For this review, take the finished solid that the model builds, in its own axes (mm). Coordinates: 2 decimals unless noted, no trailing zeros. Write each loop counter-clockwise with the first axis right and the second up, starting at its lowest first coordinate (ties: lowest second). Pieces come first, ordered by that corner, then holes. Notation, with made-up numbers: (28, -31.75) -> (40, -31.75) arc R35 cw to (40, 7.25) -> close; hole circle Ø4 at (-10, 65). An arc over 180 degrees is marked (long way). Put each result on its own line as item: value. Start each with the question number.
Item 1: Insertion check: P1, Ø1, axis at x = 56.5, y = 57, coming from the +Z side; P2, Ø2, axis at y = 45.5, z = 4.5, coming from the -X side; P3, Ø2, axis at x = -33.5, z = 5, coming from the -Y side; P4, Ø1.5, axis at y = 9.5, z = 1, coming from the +X side. Each pin has a flat end and moves straight along its axis. Give the tip position at first contact, or say it passes through.
Item 2: The part is to be moulded in two halves that separate along Y. For faces 1 (the flat face through (1, 75, 5)), 2 (the flat face through (18, 1, 0)), 3 (the cylindrical face through (75.092, 15.007, 5.055)), say which applies: +Y half, -Y half, draft (parallel to the pull), parting line (faces both ways), or undercut.
Item 3: Consider section A-A on z = 8.5. Give the boundary of the cut face in (x, y), and give its area (3 significant figures).
Item 4: Consider section B-B on x = 0. Give the boundary of the cut face in (y, z).
Item 5: To check wall thickness, follow L1, parallel to Y at x = 0, z = 4.25; L2, parallel to Y at x = -10, z = 0.5; L3, parallel to X at y = -10, z = 4.75. State the ranges of each line that lie inside material, in increasing order.
Item 6: Consider section C-C on y = -58.5. Give the boundary of the cut face in (x, z), and give its area (3 significant figures).
Item 7: Consider section D-D on x = 68. Give the boundary of the cut face in (y, z).
```python
from build123d import *

# Parameters (mm, degrees)
BOSS_EXTRUDE1_DEPTH = 10
SKETCH2_R           = 1.25
CUT_EXTRUDE1_DEPTH  = 5
CIRPATTERN1_COUNT   = 3
SKETCH3_R           = 15
CUT_EXTRUDE2_DEPTH  = 10


with BuildPart() as part:
    # Sketch1 → Boss-Extrude1 (new body)
    with BuildSketch(Plane.XY):
        Polygon((43.301270189, -75), (86.602540378, 0), (43.301270189, 75), (-43.301270189, 75), (-86.602540378, 0), (-43.301270189, -75), align=None)
    extrude(amount=BOSS_EXTRUDE1_DEPTH)

    # Sketch2 → Cut-Extrude1 (cut)
    with BuildSketch(Plane.XZ.offset(75)):
        with Locations((-33.301270189, 5)):
            Circle(SKETCH2_R)
        with Locations((-23.301270189, 5)):
            Circle(SKETCH2_R)
        with Locations(Location((33.301270189, 5, 0), (0, 0, 180))):
            Circle(SKETCH2_R)
        with Locations(Location((23.301270189, 5, 0), (0, 0, 180))):
            Circle(SKETCH2_R)
    cut_extrude1 = extrude(amount=-CUT_EXTRUDE1_DEPTH, mode=Mode.SUBTRACT)

    # CirPattern1: Cut-Extrude1 ×3 about axis
    cirpattern1_axis = Axis((0, 0, 0), (0, 0, 1))
    for i in range(1, CIRPATTERN1_COUNT):
        add(cut_extrude1.rotate(cirpattern1_axis, i * 360 / CIRPATTERN1_COUNT), mode=Mode.SUBTRACT)

    # Sketch3 → Cut-Extrude2 (cut)
    with BuildSketch(Plane.XY.offset(10)):
        Circle(SKETCH3_R)
    extrude(amount=-CUT_EXTRUDE2_DEPTH, mode=Mode.SUBTRACT)


solid = part.part
```
Return value:
1. P1: through
1. P2: x = -60.91
1. P3: y = -70
1. P4: x = 81.55
2. face 1: +Y half
2. face 2: draft
2. face 3: undercut
3. outline: (-86.6, 0) -> (-43.3, -75) -> (43.3, -75) -> (86.6, 0) -> (43.3, 75) -> (-43.3, 75) -> close; hole circle Ø30 at (0, 0)
3. area: 18,800 mm^2
4. outline: (-75, 0) -> (-15, 0) -> (-15, 10) -> (-75, 10) -> close; (15, 0) -> (75, 0) -> (75, 10) -> (15, 10) -> close
5. L1: -75 to -15, 15 to 75
5. L2: -75 to -11.18, 11.18 to 75
5. L3: -80.83 to -11.18, 11.18 to 80.83
6. outline: (-52.83, 0) -> (52.83, 0) -> (52.83, 10) -> (-52.83, 10) -> close
6. area: 1,060 mm^2
7. outline: (-32.22, 0) -> (32.22, 0) -> (32.22, 10) -> (-32.22, 10) -> close
